```python
from build123d import *

# Parameters (mm, degrees)
F1_DEPTH = 6.35
F2_DEPTH = 39.497
F3_DEPTH = 50.8
F4_R     = 2.54
F6_DEPTH = 31.75


# Not quite as in the source:
# - a fillet or chamfer that OpenCascade refuses, or shapes differently, is made with other operations: its cross-section is extruded or revolved along the edge and cut away or added


with BuildPart() as f1:
    # F0 (on Right) → F1 (new body)
    with BuildSketch(Plane.YZ):
        with BuildLine():
            Line((0, 79.1307692308), (-25.4, 79.1307692308))
            Line((-25.4, 79.1307692308), (-25.4, -79.6192307692))
            Line((-25.4, -79.6192307692), (0, -79.6192307692))
            Line((0, -79.6192307692), (0, -68.9766307692))
            ThreePointArc((0, -68.9766307692), (-2.0574, -66.9192307692), (0, -64.8618307692))
            Line((0, -64.8618307692), (0, -54.2192307692))
            Line((0, -54.2192307692), (0, -41.5192307692))
            Line((0, -41.5192307692), (0, 15.6307692308))
            ThreePointArc((0, 15.6307692308), (-12.7, 28.3307692308), (0, 41.0307692308))
            Line((0, 41.0307692308), (0, 79.1307692308))
        make_face()
        with BuildLine():
            Line((25.4, 79.1307692308), (0, 79.1307692308))
            Line((0, 79.1307692308), (0, 41.0307692308))
            ThreePointArc((0, 41.0307692308), (8.9802561211, 37.3110253518), (12.7, 28.3307692308))
            ThreePointArc((12.7, 28.3307692308), (8.9802561211, 19.3505131097), (0, 15.6307692308))
            Line((0, 15.6307692308), (0, -41.5192307692))
            Line((0, -41.5192307692), (0, -54.2192307692))
            Line((0, -54.2192307692), (0, -64.8618307692))
            ThreePointArc((0, -64.8618307692), (1.4548014916, -65.4644292776), (2.0574, -66.9192307692))
            ThreePointArc((2.0574, -66.9192307692), (1.4548014916, -68.3740322608), (0, -68.9766307692))
            Line((0, -68.9766307692), (0, -79.6192307692))
            Line((0, -79.6192307692), (25.4, -79.6192307692))
            Line((25.4, -79.6192307692), (25.4, 79.1307692308))
        make_face()
    extrude(amount=F1_DEPTH)

    # F0 (on Right) → F2 (join)
    with BuildSketch(Plane.YZ):
        with BuildLine():
            Line((0, 37.8557692308), (0, 41.0307692308))
            ThreePointArc((0, 41.0307692308), (-12.7, 28.3307692308), (0, 15.6307692308))
            Line((0, 15.6307692308), (0, 18.8057692308))
            ThreePointArc((0, 18.8057692308), (-9.525, 28.3307692308), (0, 37.8557692308))
        make_face()
        with BuildLine():
            ThreePointArc((12.7, 28.3307692308), (8.9802561211, 37.3110253518), (0, 41.0307692308))
            Line((0, 41.0307692308), (0, 37.8557692308))
            ThreePointArc((0, 37.8557692308), (6.7351920908, 35.0659613216), (9.525, 28.3307692308))
            ThreePointArc((9.525, 28.3307692308), (6.7351920908, 21.59557714), (0, 18.8057692308))
            Line((0, 18.8057692308), (0, 15.6307692308))
            ThreePointArc((0, 15.6307692308), (8.9802561211, 19.3505131097), (12.7, 28.3307692308))
        make_face()
        with BuildLine():
            Line((0, 34.6807692308), (0, 37.8557692308))
            ThreePointArc((0, 37.8557692308), (-9.525, 28.3307692308), (0, 18.8057692308))
            Line((0, 18.8057692308), (0, 21.9807692308))
            ThreePointArc((0, 21.9807692308), (-6.35, 28.3307692308), (0, 34.6807692308))
        make_face()
        with BuildLine():
            ThreePointArc((9.525, 28.3307692308), (6.7351920908, 35.0659613216), (0, 37.8557692308))
            Line((0, 37.8557692308), (0, 34.6807692308))
            ThreePointArc((0, 34.6807692308), (4.4901280605, 32.8208972913), (6.35, 28.3307692308))
            ThreePointArc((6.35, 28.3307692308), (4.4901280605, 23.8406411702), (0, 21.9807692308))
            Line((0, 21.9807692308), (0, 18.8057692308))
            ThreePointArc((0, 18.8057692308), (6.7351920908, 21.59557714), (9.525, 28.3307692308))
        make_face()
    extrude(amount=F2_DEPTH)

    # F0 (on Right) → F3 (join)
    with BuildSketch(Plane.YZ):
        with BuildLine():
            Line((0, 28.3307692308), (0, 34.6807692308))
            ThreePointArc((0, 34.6807692308), (-6.35, 28.3307692308), (0, 21.9807692308))
            Line((0, 21.9807692308), (0, 28.3307692308))
        make_face()
        with BuildLine():
            ThreePointArc((6.35, 28.3307692308), (4.4901280605, 32.8208972913), (0, 34.6807692308))
            Line((0, 34.6807692308), (0, 28.3307692308))
            Line((0, 28.3307692308), (0, 21.9807692308))
            ThreePointArc((0, 21.9807692308), (4.4901280605, 23.8406411702), (6.35, 28.3307692308))
        make_face()
    extrude(amount=F3_DEPTH)

    # F4
    f4_edges = [f1.edges().sort_by_distance(p)[0] for p in [
        (50.8, 0, 34.680769),
    ]]
    fillet(f4_edges, radius=F4_R)

    # F5: chamfer of 2.7178 x 4.2672 on 1 edges, made by hand

    # F5_s1 → F5_t2 (revolve, cut)
    with BuildSketch(Plane.XZ):
        Polygon((4.2672, -64.8618307692), (0, -62.1440307692), (0, -64.8618307692), align=None)
    revolve(axis=Axis((0, 0, -66.9192307692), (-1, 0, 0)), mode=Mode.SUBTRACT)

    # F0 (on Right) → F6 (cut)
    with BuildSketch(Plane.YZ):
        with BuildLine():
            Line((0, 34.6807692308), (0, 37.8557692308))
            ThreePointArc((0, 37.8557692308), (-9.525, 28.3307692308), (0, 18.8057692308))
            Line((0, 18.8057692308), (0, 21.9807692308))
            ThreePointArc((0, 21.9807692308), (-6.35, 28.3307692308), (0, 34.6807692308))
        make_face()
        with BuildLine():
            Line((0, 28.3307692308), (0, 34.6807692308))
            ThreePointArc((0, 34.6807692308), (-6.35, 28.3307692308), (0, 21.9807692308))
            Line((0, 21.9807692308), (0, 28.3307692308))
        make_face()
        with BuildLine():
            ThreePointArc((6.35, 28.3307692308), (4.4901280605, 32.8208972913), (0, 34.6807692308))
            Line((0, 34.6807692308), (0, 28.3307692308))
            Line((0, 28.3307692308), (0, 21.9807692308))
            ThreePointArc((0, 21.9807692308), (4.4901280605, 23.8406411702), (6.35, 28.3307692308))
        make_face()
        with BuildLine():
            ThreePointArc((9.525, 28.3307692308), (6.7351920908, 35.0659613216), (0, 37.8557692308))
            Line((0, 37.8557692308), (0, 34.6807692308))
            ThreePointArc((0, 34.6807692308), (4.4901280605, 32.8208972913), (6.35, 28.3307692308))
            ThreePointArc((6.35, 28.3307692308), (4.4901280605, 23.8406411702), (0, 21.9807692308))
            Line((0, 21.9807692308), (0, 18.8057692308))
            ThreePointArc((0, 18.8057692308), (6.7351920908, 21.59557714), (9.525, 28.3307692308))
        make_face()
    extrude(amount=F6_DEPTH, mode=Mode.SUBTRACT)


solid = f1.part
```
Input: part model. Units: mm. Frame: model coordinates. A direction names the side the tool comes from. Give positions to 0.01 mm unless a question says otherwise; leave off trailing zeros. Order: outer loops, then holes, each group sorted by start corner. A loop starts at its lowest first (then second) coordinate and runs counter-clockwise, first axis right, second up. Notation, with made-up numbers: M 41,23 L 53,23 A23 ccw 53,39 Z; hole C 41.5,22.5 d9. An arc over 180 degrees is marked long. Return JSON: item names as keys, results as strings.
1) Section query B-B on y = -17.5. Output: boundary loops of the cut face in (x, z).
Taken from the geometry:
{"outline": "M 0,-79.62 L 6.35,-79.62 L 6.35,79.13 L 0,79.13 Z"}
2) Line query: L1, parallel to Z at x = 17, y = 0; L2, parallel to X at y = -10, z = 47; L3, parallel to Y at x = 24.5, z = 33. Output: solid intervals per line, ascending. Write a range as [from, to].
Taken from the geometry:
{"L1": "z = [15.63, 18.81], [37.86, 41.03]", "L2": "x = [0, 6.35]", "L3": "y = [-11.81, -8.3], [8.3, 11.81]"}
3) Section query C-C on x = 41. Output: boundary loops of the cut face in (y, z), and give its area (3 significant figures).
Taken from the geometry:
{"outline": "C 0,28.33 d12.7", "area": "127 mm2"}
4) Section query D-D on z = -60. Output: boundary loops of the cut face in (x, y).
Taken from the geometry:
{"outline": "M 0,-25.4 L 6.35,-25.4 L 6.35,25.4 L 0,25.4 Z"}
5) Section query A-A on x = 19.5. Output: boundary loops of the cut face in (y, z) (3 decimals), and give its area (3 significant figures).
Taken from the geometry:
{"outline": "C 0,28.331 d25.4; hole C 0,28.331 d19.05", "area": "222 mm2"}
6) Contact query for flat-ended pins moving along their axis: pin 1 (12 mm diameter, centred on x = 18, z = 34, fed in from +Y); pin 2 (1 mm diameter, centred on x = 22, z = 37.5, fed in from -Y); pin 3 (3 mm diameter, centred on x = 30.5, y = 7, fed in from -Z). Output: stop coordinate, or through.
Taken from the geometry:
{"pin 1": "stops at y = 12.7", "pin 2": "stops at y = -9.28", "pin 3": "stops at z = 16.88"}
7) Mould query, pull axis Y, two halves, no side actions, for faces 4 (the face through (3, 25.4, -1)), 5 (the face through (6.35, 0, 1)), 6 (the face through (3, -25.4, 1)), 7 (the face through (31.75, 0, 28)). Classes: released by +Y, released by -Y, zero draft, split by the parting line, or undercut.
Taken from the geometry:
{"face 4": "released by +Y", "face 5": "zero draft", "face 6": "released by -Y", "face 7": "undercut"}
8) Access query for faces 1 (the face through (3, 0, -79.619)), 2 (the face through (15.65, -2.06, 19.03)), 3 (the face through (39.497, -3, 34.2)). Directions: +Z, -Z, +X, -X, +Y, -Y. A direction counts if a zero-diameter tool reaches every point of the face in a straight line with its end or side. Return the directions, or none.
Taken from the geometry:
{"face 1": "-Z, +X, -X, +Y, -Y", "face 2": "-X", "face 3": "+X"}
